Geometry: see drawing. Coordinates: mm, zero at the bounding-box minimum. Coordinates: 2 decimals unless noted, no trailing zeros. Order: outer loops, then holes, each group sorted by start corner. A loop starts at its lowest first (then second) coordinate and runs counter-clockwise, first axis right, second up. Notation, with made-up numbers: (-16, 12.25) -> (-12, 12.25) arc R27 ccw to (-12, 45.25) -> close; hole circle Ø10 at (-39, 22). An arc over 180 degrees is marked (long way). Write each question's results on one line, items separated by ' | '. Start each with the question number.
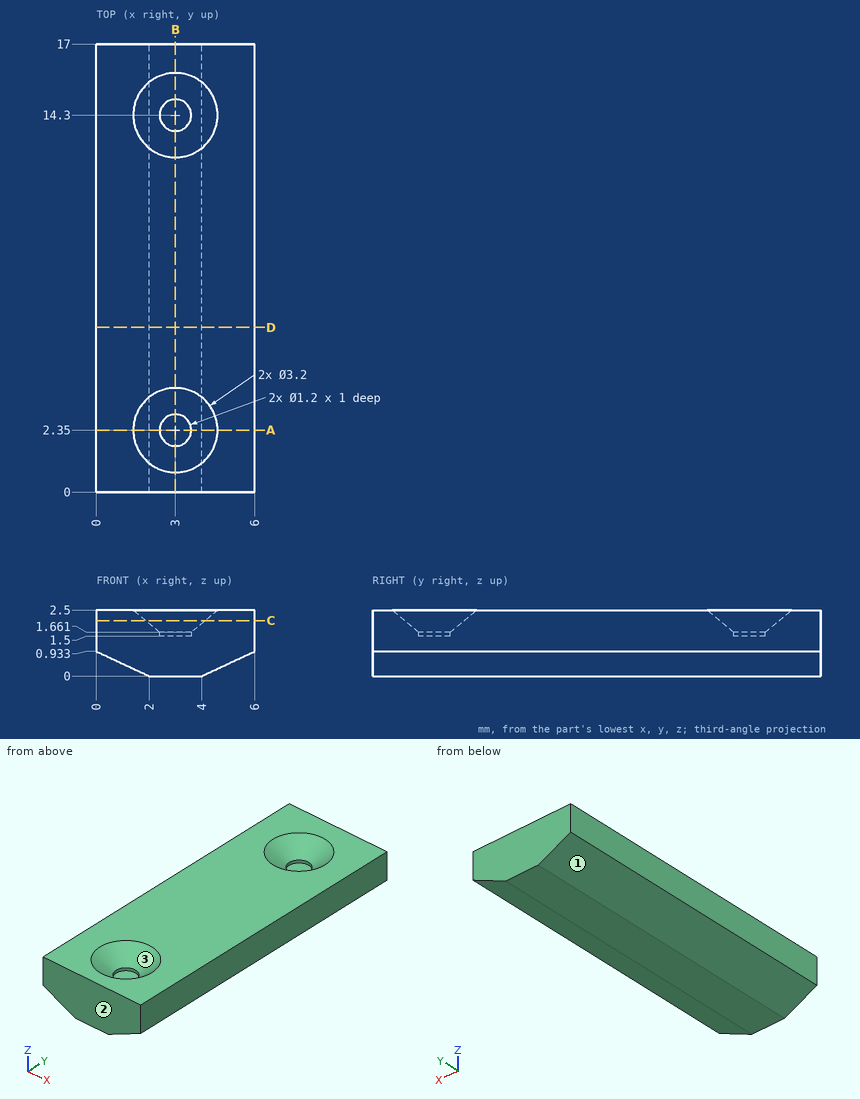
(1) Section C-C on z = 2.1. Return the cut outline in (x, y).
(2) Section B-B on x = 3. Return the cut outline in (y, z).
(3) Draft query along Y for the marked faces 1, 2 and 3. Return one class per face: released by +Y, released by -Y, zero draft, split by the parting line, or undercut.
(4) First-contact query: P1, Ø2, axis at x = 3, y = 12.5, coming from the -Z side; P2, Ø0.6, axis at x = 3, y = 14.5, coming from the +Z side; P3, Ø1.3, axis at x = 3.5, y = 2.5, coming from the +Z side; P4, Ø1.6, axis at x = 3, y = 14.3, coming from the +Z side. Flat tips, straight axial feed; report the tip coordinate or a pass-through.
(5) Line query: L1, parallel to Y at x = 3, z = 1.55; L2, parallel to X at y = 14.5, z = 2.2 (1 decimal); L3, parallel to X at y = 3, z = 2.2. Output: solid intervals per line, ascending.
(6) Section D-D on y = 6.25. Return the cut outline in (x, z).
(7) Section A-A on y = 2.35. Return the cut outline in (x, z), then the cut area to 3 significant figures.
Results list:
1) outline: (0, 0) -> (6, 0) -> (6, 17) -> (0, 17) -> close; hole circle Ø2.25 at (3, 2.35); hole circle Ø2.25 at (3, 14.3)
2) outline: (0, 0) -> (17, 0) -> (17, 2.5) -> (15.9, 2.5) -> (14.9, 1.66) -> (14.9, 1.5) -> (13.7, 1.5) -> (13.7, 1.66) -> (12.7, 2.5) -> (3.95, 2.5) -> (2.95, 1.66) -> (2.95, 1.5) -> (1.75, 1.5) -> (1.75, 1.66) -> (0.75, 2.5) -> (0, 2.5) -> close
3) face 1: zero draft | face 2: released by -Y | face 3: undercut
4) P1: stops at z = 0 | P2: stops at z = 1.5 | P3: stops at z = 2.14 | P4: stops at z = 1.83
5) L1: y = 0 to 1.75, 2.95 to 13.7, 14.9 to 17 | L2: x = 0 to 1.8, 4.2 to 6 | L3: x = 0 to 1.94, 4.06 to 6
6) outline: (0, 0.93) -> (2, 0) -> (4, 0) -> (6, 0.93) -> (6, 2.5) -> (0, 2.5) -> close
7) outline: (0, 0.93) -> (2, 0) -> (4, 0) -> (6, 0.93) -> (6, 2.5) -> (4.6, 2.5) -> (3.6, 1.66) -> (3.6, 1.5) -> (2.4, 1.5) -> (2.4, 1.66) -> (1.4, 2.5) -> (0, 2.5) -> close | area: 11.1 mm²
